Read the model definition and answer for the solid it produces. Units are mm, in the model's axes. Face numbers are marked on the shaded views. A direction names the side the tool comes from. Give positions to 0.01 mm unless a question says otherwise; leave off trailing zeros. Loops run counter-clockwise (first coordinate to the right, second up) from the corner with the lowest first, then second, coordinate; pieces in that order, holes last.
(1) Which of the six approach directions +Z, -Z, +X, -X, +Y, -Y give full straight-line access (tool end or side, diameter ignored) to the marked faces 4 and 5?
(2) Find section A-A, the plane z = 24. Write down the section's boundary in (x, y), then the cut area to 3 significant figures.
(3) Find section B-B, the plane x = -45. Write down the section's boundary in (y, z), then the cut area to 3 significant figures.
(4) This flat-tipped pin is pushed along its axis until it touches: P1, Ø4, axis at x = -15, y = 3, coming from the +Z side. Where does it stop, or does it pass through?
(5) Determine the mould class of the marked faces 1, 2 and 3 for opening direction X: pulls with the +X half, pulls with the -X half, needs draft (parallel to the pull), parting line crosses it, or undercut.
(6) Straight lines are drawn through the part: probe 1 along Y at (x, z) = (20, 24); probe 2 along Z at (x, y) = (-9, -47). For each, find the intervals that lie inside material, in ascending order.
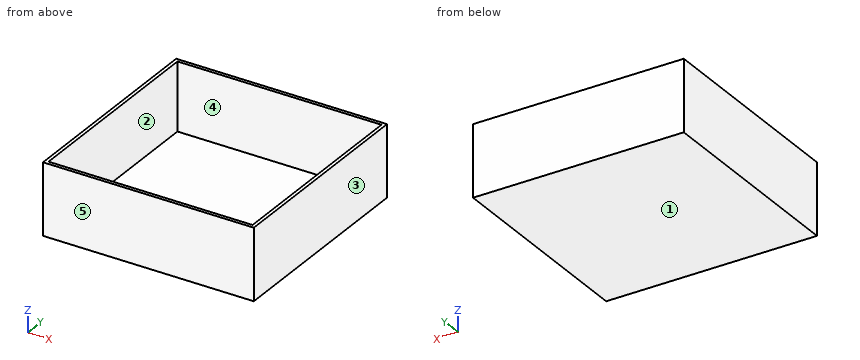
```python
from build123d import *

# Parameters (mm, degrees)
F0_W     = 124
F0_H     = 124
F0_W_2   = 120
F0_H_2   = 120
F1_DEPTH = 2
F2_DEPTH = 40


with BuildPart() as f1:
    # F0 (on Top) → F1 (new body)
    with BuildSketch(Plane.XY):
        Rectangle(F0_W, F0_H)
        Rectangle(F0_W_2, F0_H_2, mode=Mode.SUBTRACT)
        Rectangle(F0_W_2, F0_H_2)
    extrude(amount=-F1_DEPTH)

    # F0 (on Top) → F2 (join)
    with BuildSketch(Plane.XY):
        Rectangle(F0_W, F0_H)
        Rectangle(F0_W_2, F0_H_2, mode=Mode.SUBTRACT)
    extrude(amount=F2_DEPTH)


solid = f1.part
```
Entries:
1. face 4: +Z
1. face 5: +Z, -Z, +X, -X, -Y
2. outline: (-62, -62) - (62, -62) - (62, 62) - (-62, 62) - close; hole (-60, -60) - (60, -60) - (60, 60) - (-60, 60) - close
2. area: 976 mm2
3. outline: (-62, -2) - (62, -2) - (62, 40) - (60, 40) - (60, 0) - (-60, 0) - (-60, 40) - (-62, 40) - close
3. area: 408 mm2
4. P1: stops at z = 0
5. face 1: needs draft
5. face 2: undercut
5. face 3: pulls with the +X half
6. probe 1: y = -62 to -60, 60 to 62
6. probe 2: z = -2 to 0
